```python
from build123d import *

# Parameters (mm, degrees)
SKETCH2_R               = 10
BOSS_EXTRUDE1_DEPTH     = 20
CUT_EXTRUDE1_DEPTH      = 11
CUT_EXTRUDE1_DEPTH_BACK = 11
SKETCH4_R               = 3
CUT_EXTRUDE2_DEPTH      = 3


with BuildPart() as part:
    # Sketch2 → Boss-Extrude1 (new body, symmetric)
    with BuildSketch(Plane(origin=(0, 0, 0), x_dir=(1, 0, 0), z_dir=(0, 1, 0))):
        Circle(SKETCH2_R)
    extrude(amount=BOSS_EXTRUDE1_DEPTH, both=True)

    # Sketch3 → Cut-Extrude1 (cut, two sides)
    with BuildSketch(Plane.XY) as cut_extrude1_sk:
        with BuildLine():
            Line((-4.95, -7.92), (4.95, -7.92))
            Line((4.95, -7.92), (4.95, -7.095))
            ThreePointArc((4.95, -7.095), (4.845529135, -6.638488486), (4.552912235, -6.272848946))
            ThreePointArc((4.552912235, -6.272848946), (4.163263898, -4.929032869), (5.303905651, -4.118721901))
            Line((5.303905651, -4.118721901), (4.152601488, 5.595942007))
            ThreePointArc((4.152601488, 5.595942007), (2.748128038, 8.13841183), (-0.032970708, 8.976378553))
            ThreePointArc((-0.032970708, 8.976378553), (-0.420174759, 9.631170394), (-1.043370943, 10.067410979))
            Line((-1.043370943, 10.067410979), (-0.704768531, 8.852119124))
            ThreePointArc((-0.704768531, 8.852119124), (-0.961731099, 8.770731362), (-1.212370482, 8.671566707))
            Line((-1.212370482, 8.671566707), (-1.043370943, 8.000640714))
            Line((-1.043370943, 8.000640714), (-5.45370194, 4.456357119))
            ThreePointArc((-5.45370194, 4.456357119), (-5.641905535, 2.260075199), (-3.43929894, 2.172902623))
            ThreePointArc((-3.43929894, 2.172902623), (-2.20642224, 2.304167352), (-1.029214799, 2.693266345))
            Line((-1.029214799, 2.693266345), (-5.262567741, -3.352870715))
            ThreePointArc((-5.262567741, -3.352870715), (-5.32769839, -3.799977219), (-5.007467138, -4.118721901))
            ThreePointArc((-5.007467138, -4.118721901), (-4.156142001, -5.081814751), (-4.58020402, -6.295270037))
            ThreePointArc((-4.58020402, -6.295270037), (-4.853076089, -6.654455711), (-4.95, -7.095))
            Line((-4.95, -7.095), (-4.95, -7.92))
        make_face()
    extrude(amount=CUT_EXTRUDE1_DEPTH, mode=Mode.SUBTRACT)
    extrude(cut_extrude1_sk.sketch, amount=-CUT_EXTRUDE1_DEPTH_BACK, mode=Mode.SUBTRACT)

    # Sketch4 → Cut-Extrude2 (cut)
    with BuildSketch(Plane(origin=(0, -20, 0), x_dir=(-1, 0, 0), z_dir=(0, -1, 0))):
        Circle(SKETCH4_R)
    extrude(amount=-CUT_EXTRUDE2_DEPTH, mode=Mode.SUBTRACT)


solid = part.part
```
The model under review builds one solid part; all positions refer to its coordinate system, in mm. A direction names the side the tool comes from. Coordinates: 2 decimals unless noted, no trailing zeros. Loops run counter-clockwise (first coordinate to the right, second up) from the corner with the lowest first, then second, coordinate; pieces in that order, holes last. Notation, with made-up numbers: (31.5, 31.5) -> (76.5, 31.5) arc R29 ccw to (76.5, 54.5) -> close; hole circle Ø5 at (-15.75, 38). An arc over 180 degrees is marked (long way). Answer as CSV lines item,"result".
Item 1: Insertion check: pin 1 (1 mm diameter, centred on x = -1.5, y = 8.5, fed in from -Z); pin 2 (8 mm diameter, centred on x = -8, y = -11.5, fed in from -Z); pin 3 (3 mm diameter, centred on y = 11.5, z = 5, fed in from +X). Each pin has a flat end and moves straight along its axis. Give the tip position at first contact, or say it passes through.
Results below:
pin 1,"stops at z = -9.94"
pin 2,"stops at z = -9.17"
pin 3,"stops at x = 9.37"
Item 2: Take a section at D-D, the plane y = -15.5. State the section outline as (x, z) points.
Results below:
outline,"circle Ø20 at (0, 0)"
Item 3: Take a section at C-C, the plane x = -2. State the section outline as (y, z) points, and give its area (3 significant figures).
Results below:
outline,"(-20, -9.8) -> (-7.92, -9.8) -> (-7.92, 9.8) -> (-20, 9.8) -> (-20, 2.24) -> (-17, 2.24) -> (-17, -2.24) -> (-20, -2.24) -> close; (1.31, -9.8) -> (2.35, -9.8) -> (2.35, 9.8) -> (1.31, 9.8) -> close; (7.23, -9.8) -> (20, -9.8) -> (20, 9.8) -> (7.23, 9.8) -> close"
area,"494 mm2"
Item 4: Draft analysis for pull direction X (two halves, no side actions). For faces 4 (the flat face through (2.1, -20, -2.4)), 5 (the cylindrical face through (5.38, 0.28, -8.43)), 6 (the cylindrical face through (3, -19, 0)), state which applies: +X half, -X half, draft (parallel to the pull), parting line (faces both ways), or undercut.
Results below:
face 4,"draft"
face 5,"parting line"
face 6,"undercut"
Item 5: Take a section at A-A, the plane z = 0. State the section outline as (x, y) points (3 decimals), and give its area (3 significant figures).
Results below:
outline,"(-10, -20) -> (-3, -20) -> (-3, -17) -> (3, -17) -> (3, -20) -> (10, -20) -> (10, 20) -> (-10, 20) -> close; hole (-5.454, 4.456) arc R1.524 ccw (long way) to (-3.439, 2.173) arc R5.828 ccw to (-1.029, 2.693) -> (-5.263, -3.353) arc R0.503 ccw to (-5.007, -4.119) arc R1.271 cw to (-4.58, -6.295) arc R1.05 ccw to (-4.95, -7.095) -> (-4.95, -7.92) -> (4.95, -7.92) -> (4.95, -7.095) arc R1.05 ccw to (4.553, -6.273) arc R1.208 cw to (5.304, -4.119) -> (4.153, 5.596) arc R3.851 ccw to (-0.033, 8.976) arc R1.799 ccw to (-1.043, 10.067) -> (-0.705, 8.852) arc R3.851 ccw to (-1.212, 8.672) -> (-1.043, 8.001) -> close"
area,"641 mm2"
Item 6: For L1, parallel to X at y = -18.55, z = 0; L2, parallel to Y at x = 2.25, z = -2.5, list the stretches that pass through material, from the lowest coordinate up.
Results below:
L1,"x = -10 to -3, 3 to 10"
L2,"y = -20 to -7.92, 8.48 to 20"
Item 7: Take a section at B-B, the plane x = 2.5. State the section outline as (y, z) points, and give its area (3 significant figures).
Results below:
outline,"(-20, -9.68) -> (-7.92, -9.68) -> (-7.92, 9.68) -> (-20, 9.68) -> (-20, 1.66) -> (-17, 1.66) -> (-17, -1.66) -> (-20, -1.66) -> close; (8.32, -9.68) -> (20, -9.68) -> (20, 9.68) -> (8.32, 9.68) -> close"
area,"450 mm2"
Item 8: Machinability: for faces 1 (the flat face through (0, 20, 0)), 2 (the flat face through (-3.12, -0.29, 0.14)), 3 (the flat face through (0, -17, 0)), which of the approach directions +Z, -Z, +X, -X, +Y, -Y give a long, thin tool a straight path to every point of the face, cutting with its end or side? Answer none if there is none.
Results below:
face 1,"+Z, -Z, +X, -X, +Y"
face 2,"+Z, -Z"
face 3,"-Y"
